Could you check a few things on this model? Use its own coordinates, in mm. A direction names the side the tool comes from. Coordinates: 2 decimals unless noted, no trailing zeros. Order: outer loops, then holes, each group sorted by start corner. A loop starts at its lowest first (then second) coordinate and runs counter-clockwise, first axis right, second up. Notation, with made-up numbers: (-23.75, 43) -> (-14.75, 43) arc R28 cw to (-14.75, 80) -> close; hole circle Ø10 at (89, -34). An arc over 180 degrees is marked (long way). Put each result on its own line as item: value. Start each with the question number.
Q1. If we section it at C-C (y = 7.75): Please give me the cut outline in (x, z), and give its area (3 significant figures).
Q2. Please list where these lines run through material, in increasing order: line 1 along Y through (x, z) = (-9, 0.3); line 2 along Y through (x, z) = (-5.5, 1.25); line 3 along X through (y, z) = (-4.75, 1.6).
Q3. We'd pull the mould along Y, two halves only. Please class faces 5 (the face through (-9, 12.5, 1)), 6 (the face through (1, 0, 3)), 7 (the face through (0, 0, 1)): +Y half, -Y half, draft (parallel to the pull), parting line (faces both ways), or undercut.
Q4. If we section it at D-D (y = 2.75): Please give me the cut outline in (x, z), and give its area (3 significant figures).
Q5. Will these pins go through, and if not, where does the flat tip stop? pin 1 (1.2 mm diameter, centred on y = 13.5, z = 1.5, fed in from -X); pin 2 (1.5 mm diameter, centred on x = -9.5, z = 1, fed in from -Y); pin 3 (0.9 mm diameter, centred on x = -9, z = 1, fed in from +Y).
Q6. For faces 1 (the face through (-10, 9.5, 1)), 2 (the face through (-9, -12.5, 1)), 3 (the face through (-8, 13, 1)), 4 (the face through (1, 0, 0)), which set-ups out of +Z, -Z, +X, -X, +Y, -Y let a thin tool reach every point of the face, with its end or its side?
Q7. If we section it at A-A (x = -3.25): Please give me the cut outline in (y, z), and give its area (3 significant figures).
Q8. If we section it at B-B (z = 2.05): Please give me the cut outline in (x, y), and give its area (3 significant figures).
from build123d import *

# Parameters (mm, degrees)
SALIENTE_EXTRUIR1_DEPTH = 3


with BuildPart() as part:
    # Croquis1 → Saliente-Extruir1 (new body)
    with BuildSketch(Plane.XY):
        Polygon((-8, 12.5), (-11, 12.5), (-11, 9.5), (-8, 9.5), (-8, 6.5), (0, 6.5), (0, 0), (3, 0), (3, 14), (-8, 14), align=None)
    saliente_extruir1 = extrude(amount=SALIENTE_EXTRUIR1_DEPTH)

    # Simetría1: Saliente-Extruir1 across plane
    add(saliente_extruir1.mirror(Plane(origin=(0, 0, 3), x_dir=(0, 0, 1), z_dir=(0, 1, 0))))


solid = part.part
The answers:
1. outline: (-8, 0) -> (3, 0) -> (3, 3) -> (-8, 3) -> close
1. area: 33.0 mm^2
2. line 1: -12.5 to -9.5, 9.5 to 12.5
2. line 2: -14 to -6.5, 6.5 to 14
2. line 3: 0 to 3
3. face 5: +Y half
3. face 6: draft
3. face 7: undercut
4. outline: (0, 0) -> (3, 0) -> (3, 3) -> (0, 3) -> close
4. area: 9.00 mm^2
5. pin 1: x = -8
5. pin 2: y = -12.5
5. pin 3: y = 12.5
6. face 1: +Z, -Z, -X
6. face 2: +Z, -Z, -X, -Y
6. face 3: +Z, -Z, -X, +Y
6. face 4: -Z, +X, -X, +Y, -Y
7. outline: (-14, 0) -> (-6.5, 0) -> (-6.5, 3) -> (-14, 3) -> close; (6.5, 0) -> (14, 0) -> (14, 3) -> (6.5, 3) -> close
7. area: 45.0 mm^2
8. outline: (-11, -12.5) -> (-8, -12.5) -> (-8, -14) -> (3, -14) -> (3, 14) -> (-8, 14) -> (-8, 12.5) -> (-11, 12.5) -> (-11, 9.5) -> (-8, 9.5) -> (-8, 6.5) -> (0, 6.5) -> (0, -6.5) -> (-8, -6.5) -> (-8, -9.5) -> (-11, -9.5) -> close
8. area: 222 mm^2
